Design review of the part built by this model. Coordinates are the model's own, in mm. Coordinates: 2 decimals unless noted, no trailing zeros. Loops run counter-clockwise (first coordinate to the right, second up) from the corner with the lowest first, then second, coordinate; pieces in that order, holes last.
Q1. Add section D-D on x = 45. Give the boundary of the cut face in (y, z).
Q2. Add section A-A on z = 10. Give the boundary of the cut face in (x, y).
Q3. Add section B-B on x = 22.5. Give the boundary of the cut face in (y, z), and give its area (3 significant figures).
Q4. Add section C-C on y = 1.1. Give the boundary of the cut face in (x, z).
Q5. Wall thickness on probe 1 along X at (y, z) = (2.9, 10); probe 2 along X at (y, z) = (1.2, 15); probe 3 along Z at (x, y) = (45, 1.3): over which ranges is each line inside the solid? List them lowest first.
Q6. For P1, Ø3, axis at x = 45, z = 5, coming from the +Y side; P2, Ø3.5, axis at x = -22.5, z = 10, coming from the +Y side, all flat-tipped, find the tip position at first contact; note any pin that passes through.
Q7. Draft analysis for pull direction Z (two halves, no side actions). For faces 1 (the face through (-1, 0, 10)), 2 (the face through (44.792, 1.521, 13.414)), 3 (the face through (-1, 3, 20)), state which applies: released by +Z, released by -Z, zero draft, split by the parting line, or undercut.
```python
from build123d import *

# Parameters (mm, degrees)
ESQUISSE1_W                     = 100
ESQUISSE1_H                     = 20
BOSS_EXTRU_1_DEPTH              = 5
DIAM_TRE_DU_PER_AGE_3_2_3_2_1_D = 3.2
DIAM_TRE_DU_PER_AGE_3_2_3_2_2_D = 3.2
CONG_1_R                        = 1
CHANFREIN1_SIZE                 = 2
CHANFREIN2_SIZE                 = 2


with BuildPart() as part:
    # Esquisse1 → Boss.-Extru.1 (new body)
    with BuildSketch(Plane(origin=(0, 5, 0), x_dir=(1, 0, 0), z_dir=(0, 1, 0))):
        with Locations((0, -10)):
            Rectangle(ESQUISSE1_W, ESQUISSE1_H)
    extrude(amount=-BOSS_EXTRU_1_DEPTH)

    # Diamètre du perçage Ø3.2 (3.2)1 (through all)
    with Locations(Plane(origin=(0, 5, 0), x_dir=(1, 0, 0), z_dir=(0, 1, 0))):
        with Locations((22.5, -10), (-22.5, -10)):
            Hole(DIAM_TRE_DU_PER_AGE_3_2_3_2_1_D / 2)

    # Diamètre du perçage Ø3.2 (3.2)2 (through all)
    with Locations(Plane(origin=(0, 0, 0), x_dir=(-1, 0, 0), z_dir=(0, -1, 0))):
        with Locations((45, -15), (45, -5), (-45, -5), (-45, -15)):
            Hole(DIAM_TRE_DU_PER_AGE_3_2_3_2_2_D / 2)

    # Congé1
    cong_1_edges = [part.edges().sort_by_distance(p)[0] for p in [
        (-50, 2.5, 20),
        (-50, 2.5, 0),
        (50, 2.5, 0),
        (50, 2.5, 20),
    ]]
    fillet(cong_1_edges, radius=CONG_1_R)

    # Chanfrein1
    chanfrein1_edges = [part.edges().sort_by_distance(p)[0] for p in [
        (43.4, 5, 15),
        (43.4, 5, 5),
        (-46.6, 5, 5),
        (-46.6, 5, 15),
    ]]
    chamfer(chanfrein1_edges, length=CHANFREIN1_SIZE)

    # Chanfrein2
    chanfrein2_edges = [part.edges().sort_by_distance(p)[0] for p in [
        (-20.9, 0, 10),
        (24.1, 0, 10),
    ]]
    chamfer(chanfrein2_edges, length=CHANFREIN2_SIZE)


solid = part.part
```
Entries:
1. outline: (0, 0) - (5, 0) - (5, 1.4) - (3, 3.4) - (0, 3.4) - close; (0, 6.6) - (3, 6.6) - (5, 8.6) - (5, 11.4) - (3, 13.4) - (0, 13.4) - close; (0, 16.6) - (3, 16.6) - (5, 18.6) - (5, 20) - (0, 20) - close
2. outline: (-50, 0) - (-26.1, 0) - (-24.1, 2) - (-24.1, 5) - (-50, 5) - close; (-20.9, 2) - (-18.9, 0) - (18.9, 0) - (20.9, 2) - (20.9, 5) - (-20.9, 5) - close; (24.1, 2) - (26.1, 0) - (50, 0) - (50, 5) - (24.1, 5) - close
3. outline: (0, 0) - (5, 0) - (5, 8.4) - (2, 8.4) - (0, 6.4) - close; (0, 13.6) - (2, 11.6) - (5, 11.6) - (5, 20) - (0, 20) - close
3. area: 80.0 mm2
4. outline: (-50, 1) arc R1 ccw to (-49, 0) - (49, 0) arc R1 ccw to (50, 1) - (50, 19) arc R1 ccw to (49, 20) - (-49, 20) arc R1 ccw to (-50, 19) - close; hole circle Ø3.2 at (-45, 5); hole circle Ø3.2 at (-45, 15); hole circle Ø5 at (-22.5, 10); hole circle Ø5 at (22.5, 10); hole circle Ø3.2 at (45, 5); hole circle Ø3.2 at (45, 15)
5. probe 1: x = -50 to -24.1, -20.9 to 20.9, 24.1 to 50
5. probe 2: x = -50 to -46.6, -43.4 to 43.4, 46.6 to 50
5. probe 3: z = 0 to 3.4, 6.6 to 13.4, 16.6 to 20
6. P1: passes through
6. P2: stops at y = 5
7. face 1: zero draft
7. face 2: undercut
7. face 3: released by +Z
